Part model, mm, in its own coordinate system. A direction names the side the tool comes from. Round coordinates to 2 decimals unless told otherwise and drop trailing zeros. Write each loop counter-clockwise with the first axis right and the second up, starting at its lowest first coordinate (ties: lowest second). Pieces come first, ordered by that corner, then holes.
```python
from build123d import *

# Parameters (mm, degrees)
SKETCH_1_R          = 5
SKETCH_1_R_2        = 15
SKETCH_1_R_3        = 1.5
EXTRUDE_1_DEPTH     = 5
CUT_EXTRUDE_1_DEPTH = 75.498322129
FILLET_1_R          = 2
FILLET_2_R          = 5


with BuildPart() as part:
    # 草图1 → 凸台-拉伸1 (new body)
    with BuildSketch(Plane(origin=(0, 0, 0), x_dir=(1, 0, 0), z_dir=(0, 1, 0))):
        with BuildLine():
            Line((-10, 0), (-10, 22.087121525))
            ThreePointArc((-10, 22.087121525), (0, 70), (10, 22.087121525))
            Line((10, 22.087121525), (10, 0))
            ThreePointArc((10, 0), (0, -10), (-10, 0))
        make_face()
        with Locations(Location((0, 0, 0), (0, 0, 270))):
            Circle(SKETCH_1_R, mode=Mode.SUBTRACT)
        with Locations(Location((0, 45, 0), (0, 0, 270))):
            Circle(SKETCH_1_R_2, mode=Mode.SUBTRACT)
        with Locations(Location((0, 65, 0), (0, 0, 270))):
            Circle(SKETCH_1_R_3, mode=Mode.SUBTRACT)
        with Locations(Location((17.320508076, 35, 0), (0, 0, 270))):
            Circle(SKETCH_1_R_3, mode=Mode.SUBTRACT)
        with Locations(Location((-17.320508076, 35, 0), (0, 0, 270))):
            Circle(SKETCH_1_R_3, mode=Mode.SUBTRACT)
    extrude(amount=EXTRUDE_1_DEPTH)

    # 草图2 → 切除-拉伸1 (cut, through all)
    with BuildSketch(Plane(origin=(0, 5, 0), x_dir=(1, 0, 0), z_dir=(0, 1, 0))):
        with BuildLine():
            ThreePointArc((5, 20.505102572), (0, 20), (-5, 20.505102572))
            Line((-5, 20.505102572), (-5, 8.660254038))
            ThreePointArc((-5, 8.660254038), (0, 10), (5, 8.660254038))
            Line((5, 8.660254038), (5, 20.505102572))
        make_face()
    extrude(amount=-CUT_EXTRUDE_1_DEPTH, mode=Mode.SUBTRACT)

    # 圆角1
    fillet_1_edges = [part.edges().sort_by_distance(p)[0] for p in [
        (5, 2.5, -8.660254038),
        (-5, 2.5, -8.660254038),
        (-5, 2.5, -20.505102572),
        (5, 2.5, -20.505102572),
    ]]
    fillet(fillet_1_edges, radius=FILLET_1_R)

    # 圆角2
    fillet_2_edges = [part.edges().sort_by_distance(p)[0] for p in [
        (10, 2.5, -22.087121525),
        (-10, 2.5, -22.087121525),
    ]]
    fillet(fillet_2_edges, radius=FILLET_2_R)


solid = part.part
```
Q1. Cut at D-D on y = 1.25. Write the cut outline in (x, z).
Values follow:
outline: (-12.5, -23.35) arc R25 ccw (long way) to (12.5, -23.35) arc R5 cw to (10, -19.02) - (10, 0) arc R10 ccw to (-10, 0) - (-10, -19.02) arc R5 cw to start; hole circle Ø3 at (-17.32, -35); hole circle Ø30 at (0, -45); hole (-5, -18.17) arc R2 ccw to (-2.78, -20.15) arc R25 cw to (2.78, -20.15) arc R2 ccw to (5, -18.17) - (5, -11.62) arc R2 ccw to (2.5, -9.68) arc R10 cw to (-2.5, -9.68) arc R2 ccw to (-5, -11.62) - close; hole circle Ø10 at (0, 0); hole circle Ø3 at (0, -65); hole circle Ø3 at (17.32, -35)
Q2. Drop flat-ended pins along their axis: pin 1 (1.5 mm diameter, centred on y = 2.5, z = 0.5, fed in from -X); pin 2 (3 mm diameter, centred on x = -6.5, y = 3, fed in from +Z); pin 3 (2 mm diameter, centred on x = 10.5, y = 3, fed in from -Z). Give the stop position or say it passes through.
Values follow:
pin 1: stops at x = -10
pin 2: stops at z = 8.66
pin 3: stops at z = -68.12
Q3. Cut at B-B on x = 0. Write the cut outline in (y, z), plus the area to 3 significant figures.
Values follow:
outline: (0, -70) - (5, -70) - (5, -66.5) - (0, -66.5) - close; (0, -63.5) - (5, -63.5) - (5, -60) - (0, -60) - close; (0, -30) - (5, -30) - (5, -20) - (0, -20) - close; (0, -10) - (5, -10) - (5, -5) - (0, -5) - close; (0, 5) - (5, 5) - (5, 10) - (0, 10) - close
area: 135 mm2
Q4. Cut at C-C on z = -35. Write the cut outline in (x, y).
Values follow:
outline: (-22.91, 0) - (-18.82, 0) - (-18.82, 5) - (-22.91, 5) - close; (-15.82, 0) - (-11.18, 0) - (-11.18, 5) - (-15.82, 5) - close; (11.18, 0) - (15.82, 0) - (15.82, 5) - (11.18, 5) - close; (18.82, 0) - (22.91, 0) - (22.91, 5) - (18.82, 5) - close
Q5. Wall check: L1, parallel to Z at x = 1, y = 3.4; L2, parallel to X at y = 1.15, z = -65; L3, parallel to X at y = 4.4, z = -66. Give the ranges that are in metal, low to high.
Values follow:
L1: z = -69.98 to -66.12, -63.88 to -59.97, -30.03 to -20.02, -9.95 to -4.9, 4.9 to 9.95
L2: x = -15 to -1.5, 1.5 to 15
L3: x = -13.56 to -1.12, 1.12 to 13.56
Q6. Mould opens along Z. For faces 4 (the cylindrical face through (0, 2, 10)), 5 (the flat face through (-10, 2, -9)), 6 (the cylindrical face through (4.24, 2.46, -10.05)) say: +Z half, -Z half, draft (parallel to the pull), parting line (faces both ways), or undercut.
Values follow:
face 4: +Z half
face 5: draft
face 6: undercut
Q7. Which spindle directions (+Z, -Z, +X, -X, +Y, -Y) get a long thin tool onto all of the face, cutting with end or side? Do faces 1 (the flat face through (-5.2, 5, -30.6)), 2 (the cylindrical face through (4.32, 2.46, -19.67)), 3 (the flat face through (10, 2, -10)). Say none if no direction does.
Values follow:
face 1: +Z, -Z, +X, -X, +Y
face 2: +Y, -Y
face 3: +Z, +X, +Y, -Y
Q8. Cut at A-A on z = -45. Write the cut outline in (x, y), plus the area to 3 significant figures.
Values follow:
outline: (-25, 0) - (-15, 0) - (-15, 5) - (-25, 5) - close; (15, 0) - (25, 0) - (25, 5) - (15, 5) - close
area: 100 mm2
